Check sheet for the modelled part. Datum: model origin and axes. Units: mm. A direction names the side the tool comes from. Give positions to 0.01 mm unless a question says otherwise; leave off trailing zeros. Loops run counter-clockwise (first coordinate to the right, second up) from the corner with the lowest first, then second, coordinate; pieces in that order, holes last. Notation, with made-up numbers: M -12,84.25 L 13,84.25 A19 ccw 13,108.25 Z; hole C 37,-32 d3. An arc over 180 degrees is marked long. Put each result on its own line as item: value. Start each with the question number.
```python
from build123d import *

# Parameters (mm, degrees)
BOSS_EXTRUDE1_DEPTH = 173.478
BOSS_EXTRUDE2_DEPTH = 16.522
SKETCH5_W           = 256
SKETCH5_H           = 98.478
CUT_EXTRUDE3_DEPTH  = 10
SKETCH7_R           = 5
CUT_EXTRUDE4_DEPTH  = 404.448315513


with BuildPart() as part:
    # Sketch1 → Boss-Extrude1 (new body)
    with BuildSketch(Plane.XY):
        Polygon((-103.1895488, 0), (103.1895488, 0), (128, -16.432610434), (128, -40.962966098), (118.774155672, -45.61934731), (118.774155672, -97.61934731), (126.583328469, -102.791566604), (119.25400561, -106.490753372), (119.25400561, -158.490753372), (127.063178407, -163.662972666), (119.733855548, -167.362159434), (119.733855548, -219.362159434), (128, -224.837043001), (128, -242.345271931), (101.558790198, -256), (-101.558790198, -256), (-128, -242.345271931), (-128, -224.837043001), (-119.733855548, -219.362159434), (-119.733855548, -167.362159434), (-127.063178407, -163.662972666), (-119.25400561, -158.490753372), (-119.25400561, -106.490753372), (-126.583328469, -102.791566604), (-118.774155672, -97.61934731), (-118.774155672, -45.61934731), (-128, -40.962966098), (-128, -16.432610434), align=None)
    extrude(amount=BOSS_EXTRUDE1_DEPTH)

    # Sketch3 → Boss-Extrude2 (add)
    with BuildSketch(Plane.XY.offset(173.478)):
        with BuildLine():
            Line((-109.25400561, -30.77642723), (-109.25400561, -233.134965715))
            ThreePointArc((-109.25400561, -233.134965715), (-107.53617684, -237.28217123), (-103.388971325, -239))
            Line((-103.388971325, -239), (103.388971325, -239))
            ThreePointArc((103.388971325, -239), (107.53617684, -237.28217123), (109.25400561, -233.134965715))
            Line((109.25400561, -233.134965715), (109.25400561, -32.174007784))
            ThreePointArc((109.25400561, -32.174007784), (108.447882002, -27.049094521), (104.25400561, -23.99524907))
            Line((104.25400561, -23.99524907), (104.25400561, -231.784495248))
            ThreePointArc((104.25400561, -231.784495248), (104.136715259, -232.916299233), (103.789829206, -234))
            Line((103.789829206, -234), (-101.829987525, -234))
            ThreePointArc((-101.829987525, -234), (-103.544027151, -233.290021541), (-104.25400561, -231.575981915))
            Line((-104.25400561, -231.575981915), (-104.25400561, -23.99524907))
            ThreePointArc((-104.25400561, -23.99524907), (-107.868861491, -26.563815889), (-109.25400561, -30.77642723))
        make_face()
    extrude(amount=BOSS_EXTRUDE2_DEPTH)

    # Sketch5 → Cut-Extrude3 (cut)
    with BuildSketch(Plane(origin=(0, 0, 0), x_dir=(1, 0, 0), z_dir=(0, 1, 0))):
        with Locations((0, -94.239)):
            Rectangle(SKETCH5_W, SKETCH5_H)
    extrude(amount=-CUT_EXTRUDE3_DEPTH, mode=Mode.SUBTRACT)

    # Sketch7 → Cut-Extrude4 (cut, through all)
    with BuildSketch(Plane(origin=(119.25400561, 0, 0), x_dir=(0, 0, -1), z_dir=(1, 0, 0))):
        with Locations(Location((-86.739, -132.490753372, 0), (0, 0, 90))):
            Circle(SKETCH7_R)
    extrude(amount=-CUT_EXTRUDE4_DEPTH, mode=Mode.SUBTRACT)


solid = part.part
```
Q1. Section check D-D, the plane y = -58. Record the cut outline in (x, z), then the cut area to 3 significant figures.
Q2. Mould release check, pull along Y, two halves, no side actions. Record for faces 4 (the face through (104.254, -126, 182)), 5 (the face through (123, -104.6, 85.5)), 6 (the face through (-118.53, -10.16, 85.52)): pulls with the +Y half, pulls with the -Y half, needs draft (parallel to the pull), parting line crosses it, or undercut.
Q3. Thickness scan on line 1 along Z through (x, y) = (20, -205); line 2 along Y through (x, z) = (91.5, 97); line 3 along Y through (x, z) = (-109.5, 88.5). Record the ranges inside material, lowest first. Write a range as [from, to].
Q4. Access from +Z, -Z, +X, -X, +Y, -Y to the whole of each face (thin tool, end or side, straight path). Record for faces 1 (the face through (-118.774, -72, 86)), 2 (the face through (-1, -239, 182)), 3 (the face through (122.624, -100.169, 85.525)).
Q5. Section check A-A, the plane y = -192. Record the cut outline in (x, z), then the cut area to 3 significant figures.
Q6. Section check B-B, the plane z = 49.5. Record the cut outline in (x, y).
Q7. Section check C-C, the plane x = -35.5. Record the cut outline in (y, z).
Q8. Depth check by flat-ended pin: P1, Ø13, axis at y = -92, z = 183.5, coming from the -X side; P2, Ø1.5, axis at x = -29, z = 134.5, coming from the +Y side; P3, Ø8, axis at y = -52.5, z = 159, coming from the -X side. Enter the tip coordinate at first touch or a pass-through.
Found:
1. outline: M -118.77,0 L 118.77,0 L 118.77,173.48 L 109.25,173.48 L 109.25,190 L 104.25,190 L 104.25,173.48 L -104.25,173.48 L -104.25,190 L -109.25,190 L -109.25,173.48 L -118.77,173.48 Z
1. area: 41,400 mm^2
2. face 4: needs draft
2. face 5: undercut
2. face 6: pulls with the +Y half
3. line 1: z = [0, 173.48]
3. line 2: y = [-256, -10]
3. line 3: y = [-251.9, -137.17], [-127.81, -10]
4. face 1: +Z, -Z, -X
4. face 2: +Z, +X, -X, -Y
4. face 3: +Z, -Z, +X
5. outline: M -119.73,0 L 119.73,0 L 119.73,173.48 L 109.25,173.48 L 109.25,190 L 104.25,190 L 104.25,173.48 L -104.25,173.48 L -104.25,190 L -109.25,190 L -109.25,173.48 L -119.73,173.48 Z
5. area: 41,700 mm^2
6. outline: M -128,-242.35 L -101.56,-256 L 101.56,-256 L 128,-242.35 L 128,-224.84 L 119.73,-219.36 L 119.73,-167.36 L 127.06,-163.66 L 119.25,-158.49 L 119.25,-106.49 L 126.58,-102.79 L 118.77,-97.62 L 118.77,-45.62 L 128,-40.96 L 128,-16.43 L 118.29,-10 L -118.29,-10 L -128,-16.43 L -128,-40.96 L -118.77,-45.62 L -118.77,-97.62 L -126.58,-102.79 L -119.25,-106.49 L -119.25,-158.49 L -127.06,-163.66 L -119.73,-167.36 L -119.73,-219.36 L -128,-224.84 Z
7. outline: M -256,0 L 0,0 L 0,45 L -10,45 L -10,143.48 L 0,143.48 L 0,173.48 L -234,173.48 L -234,190 L -239,190 L -239,173.48 L -256,173.48 Z; hole C -132.49,86.74 d10
8. P1: stops at x = -109.25
8. P2: stops at y = -10
8. P3: stops at x = -118.77
